Read the model definition and answer for the solid it produces. Units are mm, in the model's axes. Coordinates: 2 decimals unless noted, no trailing zeros. Loops run counter-clockwise (first coordinate to the right, second up) from the corner with the lowest first, then second, coordinate; pieces in that order, holes last. Notation, with made-up numbers: (62.25, 54) -> (117.25, 54) arc R38 cw to (117.25, 92) -> close; hole circle Ø2 at (23.25, 79.5). An arc over 180 degrees is marked (long way). Answer in a Markdown table with one row per item.
```python
from build123d import *

# Parameters (mm, degrees)
CYLINDER004_R             = 1
CYLINDER004_DEPTH         = 10
CYLINDER005_R             = 1
CYLINDER005_DEPTH         = 10
CYLINDER006_R             = 1
CYLINDER006_DEPTH         = 10
CYLINDER007_R             = 1
CYLINDER007_DEPTH         = 10
BOX003_W                  = 25.4
BOX003_H                  = 3
BOX003_DEPTH              = 17.78
FILLET_R                  = 2
FILLET001_R               = 2
FILLET002_R               = 2
FILLET003_R               = 2
FILLET003_PITCH_ANGLE     = -90
FILLET003_PLACEMENT_ANGLE = -90


with BuildPart() as cylinder004:
    # Cylinder004 → Cylinder004 (new body)
    with BuildSketch(Plane(origin=(2.54, 0, 2.54), x_dir=(1, 0, 0), z_dir=(0, -1, 0))):
        Circle(CYLINDER004_R)
    extrude(amount=CYLINDER004_DEPTH)


with BuildPart() as fusion011:
    # Cylinder005 → Cylinder005 (new body)
    with BuildSketch(Plane(origin=(2.54, 0, 15.24), x_dir=(1, 0, 0), z_dir=(0, -1, 0))):
        Circle(CYLINDER005_R)
    extrude(amount=CYLINDER005_DEPTH)

    # Fusion011: union Cylinder004
    add(cylinder004.part)


with BuildPart() as cylinder006:
    # Cylinder006 → Cylinder006 (new body)
    with BuildSketch(Plane(origin=(2.54, 0, 2.54), x_dir=(1, 0, 0), z_dir=(0, -1, 0))):
        Circle(CYLINDER006_R)
    extrude(amount=CYLINDER006_DEPTH)


with BuildPart() as fusion013:
    # Cylinder007 → Cylinder007 (new body)
    with BuildSketch(Plane(origin=(2.54, 0, 15.24), x_dir=(1, 0, 0), z_dir=(0, -1, 0))):
        Circle(CYLINDER007_R)
    extrude(amount=CYLINDER007_DEPTH)

    # Fusion012: union Cylinder006
    add(cylinder006.part)


with BuildPart() as fusion013_1:
    # Fusion012 placement: moved
    add(fusion013.part.moved(Location((20.32, 0, 0))))

    # Fusion013: union Fusion011
    add(fusion011.part)


with BuildPart() as fusion013_2:
    # Fusion013 placement: moved
    add(fusion013_1.part.moved(Location((0, 3, 0))))


with BuildPart() as obj1:
    # Box003 → Box003 (new body)
    with BuildSketch(Plane.XY):
        with Locations((12.7, 1.5)):
            Rectangle(BOX003_W, BOX003_H)
    extrude(amount=BOX003_DEPTH)

    # Cut: cut Fusion013
    add(fusion013_2.part, mode=Mode.SUBTRACT)

    # Fillet
    fillet_edges = [obj1.edges().sort_by_distance(p)[0] for p in [
        (0, 1.5, 17.78),
    ]]
    fillet(fillet_edges, radius=FILLET_R)

    # Fillet001
    fillet001_edges = [obj1.edges().sort_by_distance(p)[0] for p in [
        (0, 1.5, 0),
    ]]
    fillet(fillet001_edges, radius=FILLET001_R)

    # Fillet002
    fillet002_edges = [obj1.edges().sort_by_distance(p)[0] for p in [
        (25.4, 1.5, 0),
    ]]
    fillet(fillet002_edges, radius=FILLET002_R)

    # Fillet003
    fillet003_edges = [obj1.edges().sort_by_distance(p)[0] for p in [
        (25.4, 1.5, 17.78),
    ]]
    fillet(fillet003_edges, radius=FILLET003_R)


with BuildPart() as obj1_1:
    # Fillet003 pitch: moved
    add(obj1.part.rotate(Axis((0, 0, 0), (0, 1, 0)), FILLET003_PITCH_ANGLE))


with BuildPart() as obj1_2:
    # Fillet003 placement: moved
    add(obj1_1.part.moved(Location((71, -17.75, -5))).rotate(Axis((71, -17.75, -5), (0, 0, 1)), FILLET003_PLACEMENT_ANGLE))


solid = obj1_2.part
```
1. The mould has two halves that part along Z. Classify faces 1 (the cylindrical face through (72.521, -2.893, 18.784)), 2 (the cylindrical face through (72.52, -14.37, 18.4)), 3 (the cylindrical face through (72.52, -17.18, 19.8)), 4 (the cylindrical face through (72.52, -17.15, -4.43)): pulls with the +Z half, pulls with the -Z half, needs draft (parallel to the pull), parting line crosses it, or undercut.
A:
| item | result |
|---|---|
| face 1 | undercut |
| face 2 | undercut |
| face 3 | pulls with the +Z half |
| face 4 | pulls with the -Z half |
2. A cutting plane is placed at A-A on y = -2.51. Give the vertices of the cut face in (x, z).
A:
| item | result |
|---|---|
| outline | (71, -5) -> (74, -5) -> (74, -3.46) -> (71, -3.46) -> close; (71, -1.46) -> (74, -1.46) -> (74, 16.86) -> (71, 16.86) -> close; (71, 18.86) -> (74, 18.86) -> (74, 20.4) -> (71, 20.4) -> close |
3. A cutting plane is placed at B-B on z = 17.86. Give the vertices of the cut face in (x, y).
A:
| item | result |
|---|---|
| outline | (71, -17.75) -> (74, -17.75) -> (74, -16.21) -> (71, -16.21) -> close; (71, -14.21) -> (74, -14.21) -> (74, -3.51) -> (71, -3.51) -> close; (71, -1.51) -> (74, -1.51) -> (74, 0.03) -> (71, 0.03) -> close |
4. Given pin 1 Ø2.5 at (y, z) = (-15.21, -2.46) entering from +X, flat-ended and moving along its own axis, determine where the tip first touches the part or whether it passes through.
A:
| item | result |
|---|---|
| pin 1 | stops at x = 74 |
5. Find the intervals of material crossed by probe 1 along Y at (x, z) = (72.2, -2.46); probe 2 along Z at (x, y) = (73.3, -15.21); probe 3 along Z at (x, y) = (73.45, -14.5), in increasing order.
A:
| item | result |
|---|---|
| probe 1 | y = -17.75 to -16.21, -14.21 to -3.51, -1.51 to 0.03 |
| probe 2 | z = -5 to -3.46, -1.46 to 16.86, 18.86 to 20.4 |
| probe 3 | z = -5 to -3.16, -1.76 to 17.16, 18.56 to 20.4 |
6. A cutting plane is placed at C-C on x = 72.9. Give the vertices of the cut face in (y, z), and give its area (3 significant figures).
A:
| item | result |
|---|---|
| outline | (-17.75, -3) arc R2 ccw to (-15.75, -5) -> (-1.97, -5) arc R2 ccw to (0.03, -3) -> (0.03, 18.4) arc R2 ccw to (-1.97, 20.4) -> (-15.75, 20.4) arc R2 ccw to (-17.75, 18.4) -> close; hole circle Ø2 at (-15.21, -2.46); hole circle Ø2 at (-15.21, 17.86); hole circle Ø2 at (-2.51, -2.46); hole circle Ø2 at (-2.51, 17.86) |
| area | 436 mm2 |
